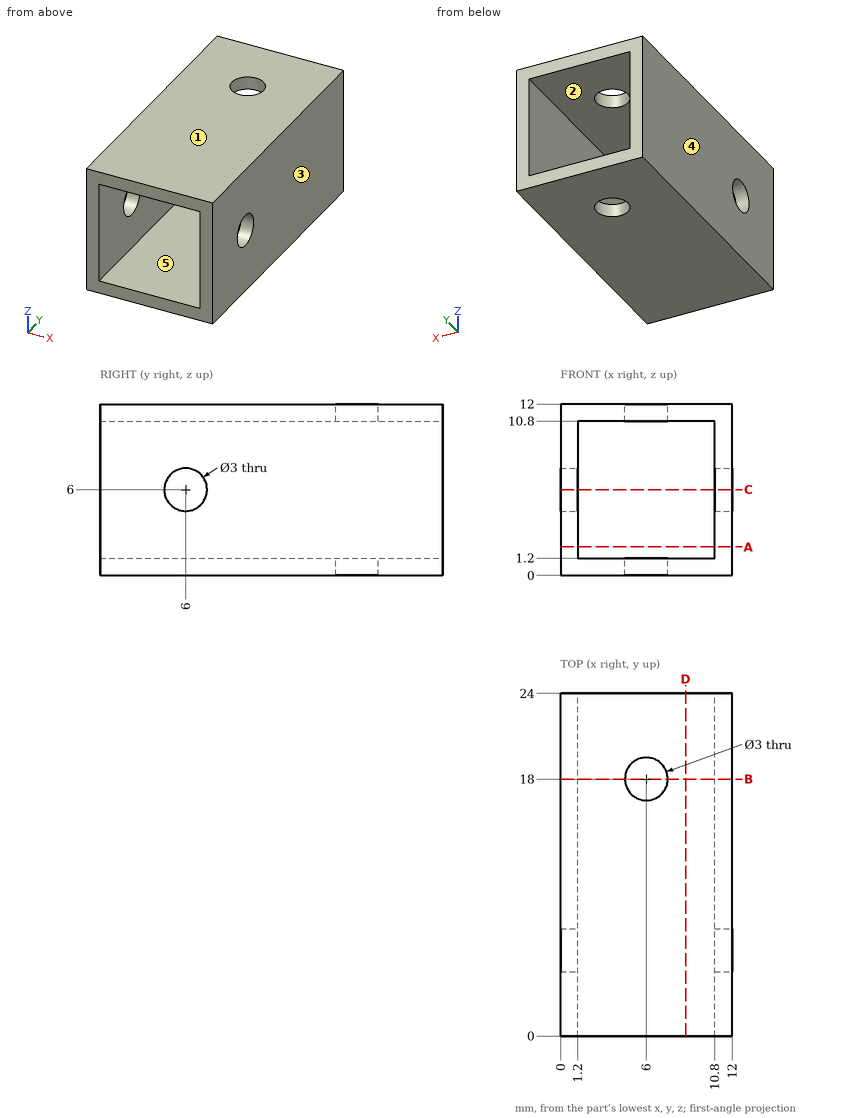
Geometry: see drawing. Coordinates: mm, zero at the bounding-box minimum. A direction names the side the tool comes from. Round coordinates to 2 decimals unless told otherwise and drop trailing zeros. Loops run counter-clockwise (first coordinate to the right, second up) from the corner with the lowest first, then second, coordinate; pieces in that order, holes last. Notation, with made-up numbers: (-0.75, 19) - (26.25, 19) arc R26 ccw to (26.25, 42) - close; hole circle Ø3 at (-35.5, -7.75). An arc over 180 degrees is marked (long way). Write item = value, one per line. Start each with the question number.
(1) Section query A-A, the plane z = 2. Output: boundary loops of the cut face in (x, y).
(2) Ray query, line 1 along X through (y, z) = (13.25, 4); line 2 along X through (y, z) = (18, 11.2). Return the intervals inside material, ascending. Write a range as from..to.
(3) Pin query (flat end, axial travel): pin 1 (1 mm diameter, centred on x = 6, z = 3, fed in from -Y); pin 2 (3.5 mm diameter, centred on x = 6, y = 18, fed in from -Z). Return the tip coordinate at first contact, or that it passes through.
(4) Section query B-B, the plane y = 18. Output: boundary loops of the cut face in (x, z), plus the area to 3 significant figures.
(5) Section query C-C, the plane z = 6. Output: boundary loops of the cut face in (x, y), plus the area to 3 significant figures.
(6) Section query D-D, the plane x = 8.75. Output: boundary loops of the cut face in (y, z).
(7) Set-up query: the marked faces 4 and 5. Return all of +Z, -Z, +X, -X, +Y, -Y with unobstructed straight access to the full face (end or side cutting, diameter ignored); none if empty.
(8) Pull-direction query (Z, two-part tool) for the marked faces 1, 2 and 3; classes: +Z half, -Z half, draft (parallel to the pull), parting line (faces both ways), or undercut.
Conclusion:
q1.outline = (0, 0) - (1.2, 0) - (1.2, 24) - (0, 24) - close; (10.8, 0) - (12, 0) - (12, 24) - (10.8, 24) - close
q2.line_1 = 0..1.2, 10.8..12
q2.line_2 = 0..4.5, 7.5..12
q3.pin_1 = through
q3.pin_2 = 0
q4.outline = (0, 0) - (4.5, 0) - (4.5, 1.2) - (1.2, 1.2) - (1.2, 10.8) - (4.5, 10.8) - (4.5, 12) - (0, 12) - close; (7.5, 0) - (12, 0) - (12, 12) - (7.5, 12) - (7.5, 10.8) - (10.8, 10.8) - (10.8, 1.2) - (7.5, 1.2) - close
q4.area = 44.6 mm2
q5.outline = (0, 0) - (1.2, 0) - (1.2, 4.5) - (0, 4.5) - close; (0, 7.5) - (1.2, 7.5) - (1.2, 24) - (0, 24) - close; (10.8, 0) - (12, 0) - (12, 4.5) - (10.8, 4.5) - close; (10.8, 7.5) - (12, 7.5) - (12, 24) - (10.8, 24) - close
q5.area = 50.4 mm2
q6.outline = (0, 0) - (24, 0) - (24, 1.2) - (0, 1.2) - close; (0, 10.8) - (24, 10.8) - (24, 12) - (0, 12) - close
q7.face_4 = +Z, -Z, -X, +Y, -Y
q7.face_5 = +Y, -Y
q8.face_1 = +Z half
q8.face_2 = undercut
q8.face_3 = draft
